Autodesk Inventor part; units mm, degrees
ref_plane "YZ Plane" through (0, 0, 0) normal (1, 0, 0) x (0, 1, 0)
ref_plane "XZ Plane" through (0, 0, 0) normal (0, 1, 0) x (-1, 0, 0)
ref_plane "XY Plane" through (0, 0, 0) normal (0, 0, 1) x (1, 0, 0)
sketch "スケッチ1" plane through (0, 0, 0) normal (0, 0, 1) x (1, 0, 0)
  line L0 (-19.75, 10) -> (19.75, 10) construction
  line L1 (19.75, 10) -> (19.75, -10) construction
  line L2 (19.75, -10) -> (-19.75, -10) construction
  line L3 (-19.75, -10) -> (-19.75, 10) construction
  line L4 (-19.75, 10) -> (19.75, -10) construction
  line L5 (19.75, 10) -> (-19.75, -10) construction
  line L6 (-19.75, 5) -> (-21.75, 5)
  line L7 (-21.75, 5) -> (-21.75, -5)
  line L8 (-19.75, 0) -> (19.75, 0) construction
  line L9 (0, 10) -> (0, -10) construction
  circle A0 centre (0, 0) radius 2.25
  arc A1 (-19.75, 5) -> (-19.75, 7.1) centre (-19.75, 6.05) ccw
  line L10 (-16.75, 10) -> (-11.75, 3)
  line L11 (-19.75, -5) -> (-21.75, -5)
  arc A2 (-19.75, -7.1) -> (-19.75, -5) centre (-19.75, -6.05) ccw
  line L12 (-16.75, -10) -> (-11.75, -3)
  line L13 (-19.75, 7.1) -> (-19.75, 10)
  line L14 (-16.75, 10) -> (-19.75, 10)
  line L15 (-16.75, -10) -> (-19.75, -10)
  line L16 (-19.75, -7.1) -> (-19.75, -10)
  line L17 (19.75, 5) -> (21.75, 5)
  line L18 (21.75, 5) -> (21.75, -5)
  arc A3 (19.75, 7.1) -> (19.75, 5) centre (19.75, 6.05) ccw
  line L19 (16.75, 10) -> (11.75, 3)
  line L20 (19.75, -5) -> (21.75, -5)
  arc A4 (19.75, -5) -> (19.75, -7.1) centre (19.75, -6.05) ccw
  line L21 (16.75, -10) -> (11.75, -3)
  line L22 (19.75, 7.1) -> (19.75, 10)
  line L23 (16.75, 10) -> (19.75, 10)
  line L24 (16.75, -10) -> (19.75, -10)
  line L25 (19.75, -7.1) -> (19.75, -10)
  arc A5 (5.1962, 3) -> (-5.1962, 3) centre (0, 0) ccw
  arc A6 (-5.1962, -3) -> (5.1962, -3) centre (0, 0) ccw
  line L26 (-1.5935, -2.76) -> (-2.1185, -1.8507) construction
  line L27 (-3.187, 0) -> (-2.662, 0.9093) construction
  line L28 (-1.5935, 2.76) -> (-0.5435, 2.76) construction
  line L29 (1.5935, 2.76) -> (2.1185, 1.8507) construction
  line L30 (3.187, 0) -> (2.662, -0.9093) construction
  line L31 (1.5935, -2.76) -> (0.5435, -2.76) construction
  arc A7 (-2.662, 0.9093) -> (-2.662, -0.9093) centre (-2.137, 0) ccw
  arc A8 (-2.1185, -1.8507) -> (-0.5435, -2.76) centre (-1.0685, -1.8507) ccw
  arc A9 (0.5435, -2.76) -> (2.1185, -1.8507) centre (1.0685, -1.8507) ccw
  arc A10 (2.662, -0.9093) -> (2.662, 0.9093) centre (2.137, 0) ccw
  arc A11 (2.1185, 1.8507) -> (0.5435, 2.76) centre (1.0685, 1.8507) ccw
  arc A12 (-0.5435, 2.76) -> (-2.1185, 1.8507) centre (-1.0685, 1.8507) ccw
  line L32 (-2.1185, 1.8507) -> (-1.5935, 2.76) construction
  line L33 (-2.662, 0.9093) -> (-2.1185, 1.8507)
  line L34 (-2.662, -0.9093) -> (-3.187, 0) construction
  line L35 (-2.1185, -1.8507) -> (-2.662, -0.9093)
  line L36 (-0.5435, -2.76) -> (-1.5935, -2.76) construction
  line L37 (0.5435, -2.76) -> (-0.5435, -2.76)
  line L38 (2.1185, -1.8507) -> (1.5935, -2.76) construction
  line L39 (2.662, -0.9093) -> (2.1185, -1.8507)
  line L40 (2.662, 0.9093) -> (3.187, 0) construction
  line L41 (2.1185, 1.8507) -> (2.662, 0.9093)
  line L42 (0.5435, 2.76) -> (1.5935, 2.76) construction
  line L43 (-0.5435, 2.76) -> (0.5435, 2.76)
  line L44 (-11.75, 3) -> (-5.1962, 3)
  line L45 (-5.1962, -3) -> (-11.75, -3)
  line L46 (5.1962, -3) -> (11.75, -3)
  line L47 (11.75, 3) -> (5.1962, 3)
  point P0 (0, 0)
  point P1 (-1.5935, -2.76)
  point P2 (1.5935, -2.76)
  point P3 (3.187, 0)
  point P4 (1.5935, 2.76)
  point P5 (-1.5935, 2.76)
  dimension "d0" = 39.5
  dimension "d3" = 4.5
  dimension "d4" = 2
  dimension "d5" = 10
  dimension "d6" = 1.05
  dimension "d7" = 3
  dimension "d9" = 5
  dimension "d11" = 8
  dimension "d12" = 6
  dimension "d14" = 1.05
  dimension "d17" = 360
  dimension "d19" = 5.52
  dimension "d20" = 6
extrude "押し出し1" add sketch "スケッチ1" along normal blind 3 contours A1 L13 L14 L10 L44 A5 L47 L19 L23 L22 A3 L17 L18 L20 A4 L25 L24 L21 L46 A6 L45 L12 L15 L16 A2 L11 L7 L6
extrude "押し出し2" add sketch "スケッチ1" along normal blind 0.8 contours L33 A12 L43 A11 L41 A10 L39 A9 L37 A8 L35 A7
fillet "フィレット1" radius 2 12 edges at (-11.75, 3, 1.5) (-11.75, -3, 1.5) (-16.75, 10, 1.5) (-16.75, -10, 1.5) (-5.1962, -3, 1.5) (-5.1962, 3, 1.5) (5.1962, 3, 1.5) (5.1962, -3, 1.5) (11.75, 3, 1.5) (11.75, -3, 1.5) (16.75, 10, 1.5) (16.75, -10, 1.5)
properties part number "Ankle_front_frame" material "アルミニウム 2014-T4"
Model file for the job. Use its own axes, mm. A direction names the side the tool comes from. Give positions to 0.01 mm unless a question says otherwise; leave off trailing zeros. Loops run counter-clockwise (first coordinate to the right, second up) from the corner with the lowest first, then second, coordinate; pieces in that order, holes last.
1) Saw through at A-A (y = 0). Write the cut outline in (x, z), plus the area to 3 significant figures.
2) Saw through at C-C (x = 9). Write the cut outline in (y, z), plus the area to 3 significant figures.
3) Pull direction X, two halves, no side cores. Call faces 5 (the cylindrical face through (-18.7, 6.1, 1.5)), 6 (the cylindrical face through (5.37, 3.2, 1.52)), 7 (the flat face through (-21, -5, 1)): +X half, -X half, draft (parallel to the pull), parting line (faces both ways), or undercut.
4) Wall check: line 1 (X direction, y = 1.75, z = 1.85); line 2 (X direction, y = -2, z = 1.25); line 3 (Y direction, x = 7, z = 0.85). Give the ranges that are in metal, low to high.
5) Saw through at B-B (x = 0). Write the cut outline in (y, z), plus the area to 3 significant figures.
6) Tool access for faces 1 (the flat face through (2.394, -1.373, 1.885)), 2 (the flat face through (-14.28, -6.54, 1.48)), 3 (the flat face through (-21, 5, 1)), 4 (the cylindrical face through (16.876, 9.784, 1.521)): list every direction of +Z, -Z, +X, -X, +Y, -Y with a clear straight run to the whole face (end or side of a thin tool).
7) Saw through at D-D (y = -6.5). Write the cut outline in (x, z).
8) Flat gauge pins, fed straight in: pin 1 Ø3.5 at (x, y) = (0, 0) entering from -Z; pin 2 Ø1.5 at (y, z) = (8.5, 1) entering from -X; pin 3 Ø1 at (x, z) = (4.5, 1.5) entering from +Y; pin 4 Ø0.6 at (x, z) = (21, 1.5) entering from -Y. Where does each tip first touch, or does it go through?
Answer block:
1. outline: (-21.75, 0) - (-2.25, 0) - (-2.25, 0.8) - (-3.19, 0.8) - (-3.19, 3) - (-21.75, 3) - close; (2.25, 0) - (21.75, 0) - (21.75, 3) - (3.19, 3) - (3.19, 0.8) - (2.25, 0.8) - close
1. area: 113 mm2
2. outline: (-3, 0) - (3, 0) - (3, 3) - (-3, 3) - close
2. area: 18.0 mm2
3. face 5: -X half
3. face 6: undercut
3. face 7: draft
4. line 1: x = -21.75 to -2.18, 2.18 to 21.75
4. line 2: x = -21.75 to -2.11, 2.11 to 21.75
4. line 3: y = -3 to 3
5. outline: (-6, 0) - (-2.25, 0) - (-2.25, 0.8) - (-2.76, 0.8) - (-2.76, 3) - (-6, 3) - close; (2.25, 0) - (6, 0) - (6, 3) - (2.76, 3) - (2.76, 0.8) - (2.25, 0.8) - close
5. area: 20.3 mm2
6. face 1: +Z
6. face 2: +Z, -Z, -Y
6. face 3: +Z, -Z, -X, +Y
6. face 4: +Z, -Z, +Y
7. outline: (-18.8, 0) - (-14.25, 0) - (-14.25, 3) - (-18.8, 3) - close; (14.25, 0) - (18.8, 0) - (18.8, 3) - (14.25, 3) - close
8. pin 1: passes through
8. pin 2: stops at x = -19.75
8. pin 3: stops at y = 4.47
8. pin 4: stops at y = -5
